Read the model definition and answer for the solid it produces. Units are mm, in the model's axes. Face numbers are marked on the shaded views. A direction names the side the tool comes from. Round coordinates to 2 decimals unless told otherwise and drop trailing zeros. Loops run counter-clockwise (first coordinate to the right, second up) from the corner with the lowest first, then second, coordinate; pieces in that order, holes last. Notation, with made-up numbers: M 26.25,-6 L 54.25,-6 A16 cw 54.25,18 Z; hole C 22,15.25 d9. An arc over 180 degrees is marked long. Write each question's results on one line, items separated by ' | '.
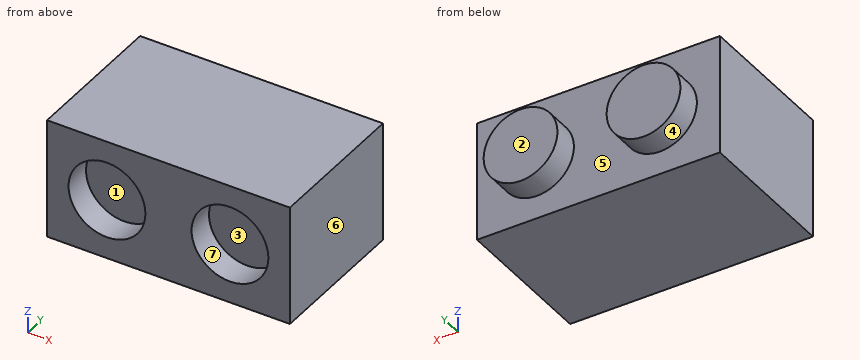
```python
from build123d import *

# Parameters (mm, degrees)
SKETCH_1_W          = 15.8
SKETCH_1_H          = 7.8
EXTRUDE_1_DEPTH     = 9.6
SKETCH_2_R          = 2.4
EXTRUDE_2_DEPTH     = 1.7
SKETCH_3_R          = 2.5
CUT_EXTRUDE_1_DEPTH = 1.8


with BuildPart() as part:
    # Эскиз1 → Бобышка-Вытянуть1 (new body)
    with BuildSketch(Plane(origin=(0, 0, 0), x_dir=(1, 0, 0), z_dir=(0, 1, 0))):
        with Locations((7.9, 3.9)):
            Rectangle(SKETCH_1_W, SKETCH_1_H)
    extrude(amount=EXTRUDE_1_DEPTH)

    # Эскиз2 → Бобышка-Вытянуть2 (add)
    with BuildSketch(Plane(origin=(0, 9.6, 0), x_dir=(1, 0, 0), z_dir=(0, 1, 0))):
        with Locations((3.9, 3.9)):
            Circle(SKETCH_2_R)
        with Locations((11.9, 3.9)):
            Circle(SKETCH_2_R)
    extrude(amount=EXTRUDE_2_DEPTH)

    # Эскиз3 → Вырез-Вытянуть1 (cut)
    with BuildSketch(Plane.XZ):
        with Locations((11.9, -3.9)):
            Circle(SKETCH_3_R)
        with Locations((3.9, -3.9)):
            Circle(SKETCH_3_R)
    extrude(amount=-CUT_EXTRUDE_1_DEPTH, mode=Mode.SUBTRACT)


solid = part.part
```
1. Find section B-B, the plane z = -3.9. Give the vertices of the cut face in (x, y).
Completed:
outline: M 0,0 L 1.4,0 L 1.4,1.8 L 6.4,1.8 L 6.4,0 L 9.4,0 L 9.4,1.8 L 14.4,1.8 L 14.4,0 L 15.8,0 L 15.8,9.6 L 14.3,9.6 L 14.3,11.3 L 9.5,11.3 L 9.5,9.6 L 6.3,9.6 L 6.3,11.3 L 1.5,11.3 L 1.5,9.6 L 0,9.6 Z
2. Determine the mould class of the marked faces 1, 2, 3 and 4 for opening direction Z: released by +Z, released by -Z, zero draft, split by the parting line, or undercut.
Completed:
face 1: undercut | face 2: zero draft | face 3: undercut | face 4: split by the parting line
3. Which of the six approach directions +Z, -Z, +X, -X, +Y, -Y give full straight-line access (tool end or side, diameter ignored) to the marked faces 5, 6 and 7?
Completed:
face 5: +Y | face 6: +Z, -Z, +X, +Y, -Y | face 7: -Y
4. Find section C-C, the plane y = 10. Give the vertices of the cut face in (x, z).
Completed:
outline: C 3.9,-3.9 d4.8; C 11.9,-3.9 d4.8
5. Find section A-A, the plane x = 11.9. Give the vertices of the cut face in (y, z), then the cut area to 3 significant figures.
Completed:
outline: M 0,-7.8 L 9.6,-7.8 L 9.6,-6.3 L 11.3,-6.3 L 11.3,-1.5 L 9.6,-1.5 L 9.6,0 L 0,0 L 0,-1.4 L 1.8,-1.4 L 1.8,-6.4 L 0,-6.4 Z | area: 74.0 mm2
6. Find the intervals of material crossed by L1, parallel to X at y = 0.75, z = -4; L2, parallel to Z at x = 11.9, y = 0.85; L3, parallel to X at y = 1.5, z = -5.25, in increasing order.
Completed:
L1: x = 0 to 1.4, 6.4 to 9.4, 14.4 to 15.8 | L2: z = -7.8 to -6.4, -1.4 to 0 | L3: x = 0 to 1.8, 6 to 9.8, 14 to 15.8
7. Find section D-D, the plane z = -5.75. Give the vertices of the cut face in (x, y).
Completed:
outline: M 0,0 L 2.22,0 L 2.22,1.8 L 5.58,1.8 L 5.58,0 L 10.22,0 L 10.22,1.8 L 13.58,1.8 L 13.58,0 L 15.8,0 L 15.8,9.6 L 13.43,9.6 L 13.43,11.3 L 10.37,11.3 L 10.37,9.6 L 5.43,9.6 L 5.43,11.3 L 2.37,11.3 L 2.37,9.6 L 0,9.6 Z
8. Given P1, Ø1.5, axis at x = 12, z = -4, coming from the -Y side, flat-ended and moving along its own axis, determine where the tip first touches the part or whether it passes through.
Completed:
P1: stops at y = 1.8
